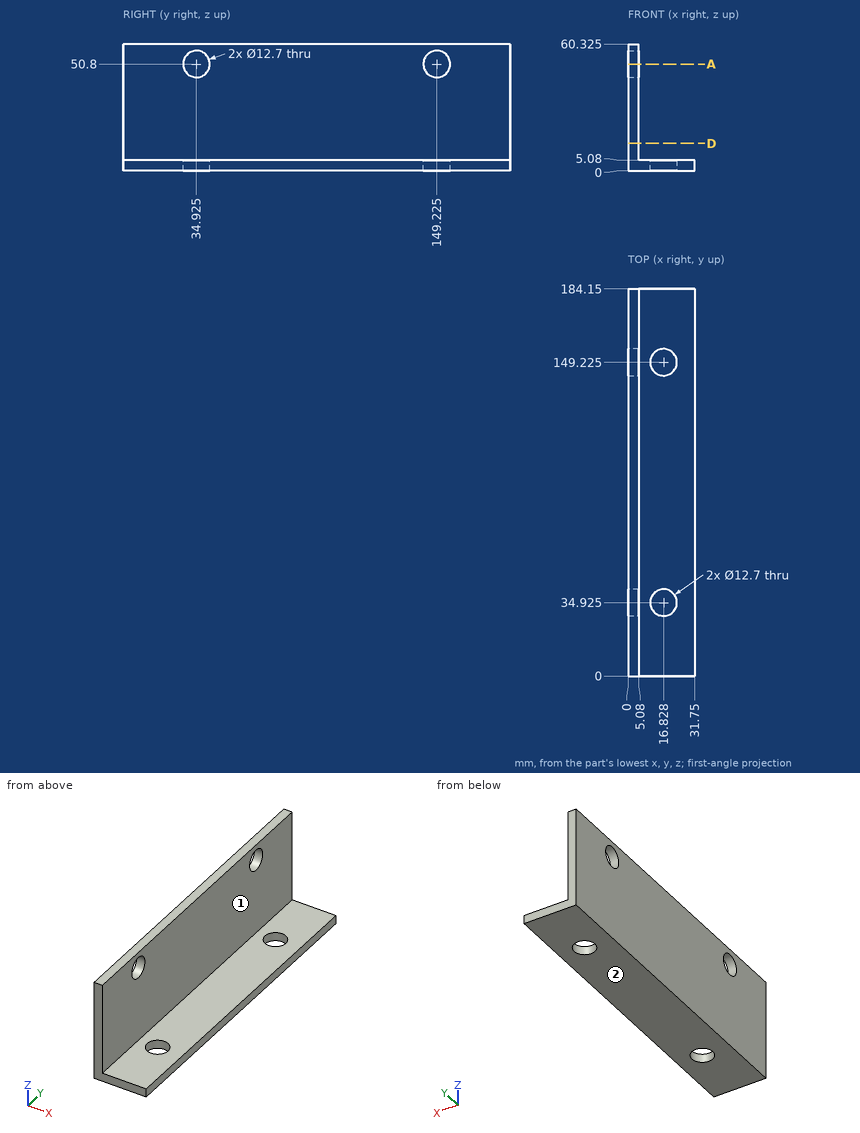
Verification items for this drawing (mm, ordinates from the low corner). A direction names the side the tool comes from. Round coordinates to 2 decimals unless told otherwise and drop trailing zeros. Loops run counter-clockwise (first coordinate to the right, second up) from the corner with the lowest first, then second, coordinate; pieces in that order, holes last. Notation, with made-up numbers: (7, -36) - (51, -36) arc R19 ccw to (51, -5) - close; hole circle Ø9 at (-18, 36). An arc over 180 degrees is marked (long way). Write item = value, one per line.
Q1. Sectioned sample at A-A on z = 50.8. State how many separate pieces and enclosed holes the cut face has.
Here are the results:
separate_pieces = 3
enclosed_holes = 0
Q2. Material ranges on L1, parallel to Z at x = 29, y = 148, recorded low to high.
Here are the results:
L1 = 0 to 5.08
Q3. Depth check by flat-ended pin: pin 1 (1.5 mm diameter, centred on y = 125.5, z = 19, fed in from +X); pin 2 (1 mm diameter, centred on x = 17.5, y = 130.5, fed in from +Z). Enter the tip coordinate at first touch or a pass-through.
Here are the results:
pin_1 = 5.08
pin_2 = 5.08
Q4. Tool access check on the marked faces 1 and 2. Record the directions out of +Z, -Z, +X, -X, +Y, -Y that give a thin tool (end or side, any length) a straight path to the whole face; none if there is none.
Here are the results:
face_1 = +Z, +X, +Y, -Y
face_2 = -Z, +X, -X, +Y, -Y
Q5. Sectioned sample at D-D on z = 13. Record the boundary of the cut face in (x, y).
Here are the results:
outline = (0, 0) - (5.08, 0) - (5.08, 184.15) - (0, 184.15) - close
